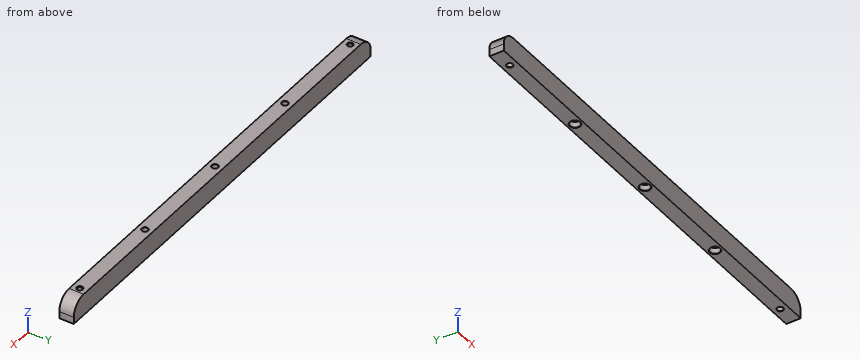
from build123d import *

# Parameters (mm, degrees)
SKETCH1_W                                    = 390.525
SKETCH1_H                                    = 19.05
EXTRUDE1_DEPTH                               = 6.35
FILLET1_R                                    = 12.954
COUNTERDRILLED_10_32_AT_2_COUNT              = 2
COUNTERDRILLED_10_32_AT_2_PITCH              = 355.6
CBORE_FOR_10_SOCKET_HEAD_CAP_SCREW1_AT_COUNT = 2
CBORE_FOR_10_SOCKET_HEAD_CAP_SCREW1_AT_PITCH = 92.075
CBORE_FOR_10_SOCKET_HEAD_CAP_SCREW1_2_COUNT  = 2
CBORE_FOR_10_SOCKET_HEAD_CAP_SCREW1_2_PITCH  = 184.15
CHAMFER1_SIZE                                = 0.254
CHAMFER2_SIZE                                = 0.5588


with BuildPart() as part:
    # Sketch1 → Extrude1 (new, symmetric)
    with BuildSketch(Plane(origin=(0, 0, 0), x_dir=(1, 0, 0), z_dir=(0, 1, 0))):
        with Locations((0, 9.525)):
            Rectangle(SKETCH1_W, SKETCH1_H)
    extrude(amount=EXTRUDE1_DEPTH, both=True)

    # Fillet1
    fillet1_edges = [part.edges().sort_by_distance(p)[0] for p in [
        (195.2625, 0, 0),
        (-195.2625, 0, 0),
    ]]
    fillet(fillet1_edges, radius=FILLET1_R)

    # Sketch3 → counterdrilled 10-32 (revolve, cut)
    with BuildSketch(Plane(origin=(177.8, 0, -19.05), x_dir=(0, 1, 0), z_dir=(1, 0, 0))):
        Polygon((0, 0), (0, 19.05), (2.0193, 19.05), (2.0193, 9.845499054), (2.5527, 9.525), (2.5527, 0), align=None)
    counterdrilled_10_32 = revolve(axis=Axis((177.8, 0, -25.180023899), (0, 0, 1)), mode=Mode.SUBTRACT)

    # counterdrilled 10-32 at 2: counterdrilled 10-32 ×2
    with Locations(*[(-i * COUNTERDRILLED_10_32_AT_2_PITCH, 0, 0) for i in range(1, COUNTERDRILLED_10_32_AT_2_COUNT)]):
        add(counterdrilled_10_32, mode=Mode.SUBTRACT)

    # Sketch5 → CBORE for #10 Socket Head Cap Screw1 (revolve, cut)
    with BuildSketch(Plane(origin=(92.075, 0, -19.05), x_dir=(0, 1, 0), z_dir=(1, 0, 0))):
        Polygon((0, 0), (0, 19.05), (2.794, 19.05), (2.5527, 18.8087), (2.5527, 5.334), (4.3688, 5.334), (4.3688, 0.254), (4.6228, 0), align=None)
    cbore_for_10_socket_head_cap_screw1 = revolve(axis=Axis((92.075, 0, -25.4), (0, 0, 1)), mode=Mode.SUBTRACT)

    # CBORE for #10 Socket Head Cap Screw1 at: CBORE for #10 Socket Head Cap Screw1 ×2
    with Locations(*[(-i * CBORE_FOR_10_SOCKET_HEAD_CAP_SCREW1_AT_PITCH, 0, 0) for i in range(1, CBORE_FOR_10_SOCKET_HEAD_CAP_SCREW1_AT_COUNT)]):
        add(cbore_for_10_socket_head_cap_screw1, mode=Mode.SUBTRACT)

    # CBORE for _10 Socket Head Cap Screw1 2: CBORE for #10 Socket Head Cap Screw1 ×2
    with Locations(*[(-i * CBORE_FOR_10_SOCKET_HEAD_CAP_SCREW1_2_PITCH, 0, 0) for i in range(1, CBORE_FOR_10_SOCKET_HEAD_CAP_SCREW1_2_COUNT)]):
        add(cbore_for_10_socket_head_cap_screw1, mode=Mode.SUBTRACT)

    # Chamfer1
    chamfer1_edges = [part.edges().sort_by_distance(p)[0] for p in [
        (-177.8, -2.5527, -19.05),
        (177.8, -2.5527, -19.05),
    ]]
    chamfer(chamfer1_edges, length=CHAMFER1_SIZE)

    # Chamfer2
    chamfer2_edges = [part.edges().sort_by_distance(p)[0] for p in [
        (-177.8, -2.0193, 0),
        (177.8, -2.0193, 0),
    ]]
    chamfer(chamfer2_edges, length=CHAMFER2_SIZE)


solid = part.part
Read the model definition and answer for the solid it produces. Units are mm, in the model's axes. Coordinates: 2 decimals unless noted, no trailing zeros. One line per question, with ' | ' between items.
Q1. Find section A-A, the plane y = 0. State how many separate pieces and enclosed holes the cut face has, plus the area to 3 significant figures.
Result set:
separate pieces: 6 | enclosed holes: 0 | area: 6,840 mm^2
Q2. Consider L1, parallel to X at y = 0, z = -14.75; L2, parallel to X at y = 0, z = -13.5; L3, parallel to Y at x = -177.8, z = -2.5. Determine where each line is inside the solid, lowest interval first. Write a range as [from, to].
Result set:
L1: [-195.26, -180.35], [-175.25, -96.44], [-87.71, -4.37], [4.37, 87.71], [96.44, 175.25], [180.35, 195.26] | L2: [-195.26, -180.35], [-175.25, -94.63], [-89.52, -2.55], [2.55, 89.52], [94.63, 175.25], [180.35, 195.26] | L3: [-6.35, -2.02], [2.02, 6.35]
Q3. Each of these flat-tipped pins is pushed along its axis until it touches: P1, Ø4.5, axis at x = 1.5, y = -0.5, coming from the -Z side; P2, Ø3.5, axis at x = -177.8, y = 0, coming from the +Z side; P3, Ø5, axis at x = -93, y = 3, coming from the -Z side; P4, Ø4.5, axis at x = -177.8, y = 0, coming from the -Z side. Where does it stop, or does it pass through?
Result set:
P1: z = -13.72 | P2: through | P3: z = -19.05 | P4: z = -9.34
